Read the model definition and answer for the solid it produces. Units are mm, in the model's axes. Face numbers are marked on the shaded views. A direction names the side the tool comes from. Coordinates: 2 decimals unless noted, no trailing zeros. Write each loop counter-clockwise with the first axis right and the second up, starting at its lowest first coordinate (ties: lowest second). Pieces come first, ordered by that corner, then holes. Notation, with made-up numbers: (35, 61) -> (88, 61) arc R23 ccw to (88, 79) -> close; hole circle Ø9 at (-17.75, -12). An arc over 180 degrees is marked (long way). Use CSV: the item, a comma, the result in double quotes.
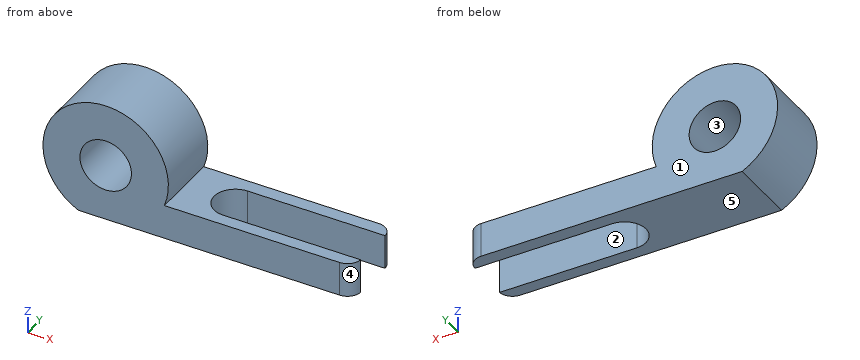
from build123d import *

# Parameters (mm, degrees)
F0_R        = 9.525
F2_DEPTH    = 25.4
F3_W        = 50.8
F3_H        = 15.748
F4_DEPTH    = 25.4
F5_T1_DEPTH = 38.0949194415
F5_T3_DEPTH = 38.0185897363


# Not quite as in the source:
# - a fillet or chamfer that OpenCascade refuses, or shapes differently, is made with other operations: its cross-section is extruded or revolved along the edge and cut away or added


with BuildPart() as f2:
    # F0 (on Front) → F2 (new body)
    with BuildSketch(Plane.XZ):
        with BuildLine():
            ThreePointArc((-20.9804001153, 12.7), (-51.2752635033, 42.3996584702), (-52.7304001153, 0))
            Line((-52.7304001153, 0), (48.8695998847, 0))
            Line((48.8695998847, 0), (48.8695998847, 12.7))
            Line((48.8695998847, 12.7), (-20.9804001153, 12.7))
        make_face()
        with Locations((-42.6671736259, 20.8794337765)):
            Circle(F0_R, mode=Mode.SUBTRACT)
    extrude(amount=F2_DEPTH)

    # F3 (on face) → F4 (cut)
    with BuildSketch(Plane.XY.offset(12.7)):
        with Locations((23.4695998847, -12.8523994962)):
            Rectangle(F3_W, F3_H)
        with BuildLine():
            ThreePointArc((-1.9304001153, -4.9783994962), (-9.8044001153, -12.8523994962), (-1.9304001153, -20.7263994962))
            Line((-1.9304001153, -20.7263994962), (-1.9304001153, -4.9783994962))
        make_face()
    extrude(amount=-F4_DEPTH, mode=Mode.SUBTRACT)

    # F5: fillet of radius 5.08 on 2 edges, made by hand

    # F5_s2 → F5_t1 (cut)
    with BuildSketch(Plane.XY.offset(-12.6974597208)):
        with BuildLine():
            ThreePointArc((43.7906159964, 0), (47.3466158165, -1.4521541819), (48.8695998847, -4.9783994962))
            Line((48.8695998847, -4.9783994962), (48.8695998847, 0))
            Line((48.8695998847, 0), (43.7906159964, 0))
        make_face()
    extrude(amount=F5_T1_DEPTH, mode=Mode.SUBTRACT)

    # F5_s4 → F5_t3 (cut)
    with BuildSketch(Plane.XY.offset(-12.6592948682)):
        with BuildLine():
            ThreePointArc((48.8695998847, -20.7263994962), (47.2513057546, -24.0530221966), (43.8058819375, -25.4))
            Line((43.8058819375, -25.4), (48.8695998847, -25.4))
            Line((48.8695998847, -25.4), (48.8695998847, -20.7263994962))
        make_face()
    extrude(amount=F5_T3_DEPTH, mode=Mode.SUBTRACT)


solid = f2.part
1. Each of these flat-tipped pins is pushed along its axis until it touches: pin 1 Ø10 at (x, z) = (-39, 37.5) entering from +Y; pin 2 Ø10 at (x, y) = (-4.5, -5) entering from +Z; pin 3 Ø6 at (y, z) = (-3, 21) entering from +X. Where does it stop, or does it pass through?
Solutions:
pin 1,"stops at y = 0"
pin 2,"stops at z = 12.7"
pin 3,"stops at x = -19.49"
2. A cutting plane is placed at B-B (z = 22). Give the vertices of the cut face in (x, y).
Solutions:
outline,"(-65.82, -25.4) -> (-52.13, -25.4) -> (-52.13, 0) -> (-65.82, 0) -> close; (-33.21, -25.4) -> (-19.52, -25.4) -> (-19.52, 0) -> (-33.21, 0) -> close"
3. For a pull along Z with two mould halves and no side action, classify the marked faces 3, 4 and 5 as pulls with the +Z half, pulls with the -Z half, needs draft (parallel to the pull), parting line crosses it, or undercut.
Solutions:
face 3,"undercut"
face 4,"needs draft"
face 5,"pulls with the -Z half"
4. A cutting plane is placed at A-A (x = 12). Give the vertices of the cut face in (y, z).
Solutions:
outline,"(-25.4, 0) -> (-20.73, 0) -> (-20.73, 12.7) -> (-25.4, 12.7) -> close; (-4.98, 0) -> (0, 0) -> (0, 12.7) -> (-4.98, 12.7) -> close"
5. A cutting plane is placed at D-D (z = 3). Give the vertices of the cut face in (x, y), and give its area (3 significant figures).
Solutions:
outline,"(-57.42, -25.4) -> (43.81, -25.4) arc R5.08 ccw to (48.87, -20.73) -> (-1.93, -20.73) arc R7.87 cw to (-1.93, -4.98) -> (48.87, -4.98) arc R5.08 ccw to (43.79, 0) -> (-57.42, 0) -> close"
area,"1,790 mm^2"
6. A tool of negligible diameter and unlimited length cuts with its end or side. For the marked faces 1 and 2, from which of +Z, -Z, +X, -X, +Y, -Y can it reach the whole face along a straight path? Write none if from no direction.
Solutions:
face 1,"+Z, -Z, +X, -X, +Y"
face 2,"+Z, -Z, +X"
7. A cutting plane is placed at C-C (y = -2). Give the vertices of the cut face in (x, z) (3 decimals).
Solutions:
outline,"(-52.73, 0) -> (47.83, 0) -> (47.83, 12.7) -> (-20.98, 12.7) arc R23.178 ccw (long way) to start; hole circle Ø19.05 at (-42.667, 20.879)"
8. Find the intervals of material crossed by line 1 along Y through (x, z) = (14.5, 5); line 2 along Z through (x, y) = (38, -23); line 3 along X through (y, z) = (-17.75, 27), in increasing order.
Solutions:
line 1,"y = -25.4 to -20.73, -4.98 to 0"
line 2,"z = 0 to 12.7"
line 3,"x = -65.02 to -49.97, -35.37 to -20.31"
